The figure shows three views and two pictorial views of one solid part (mm, origin at its lowest corner). Answer the questions. A direction names the side the tool comes from. Coordinates: 2 decimals unless noted, no trailing zeros. Loops run counter-clockwise (first coordinate to the right, second up) from the corner with the lowest first, then second, coordinate; pieces in that order, holes last. Notation, with made-up numbers: (-8.5, 81) -> (36.5, 81) arc R9 ccw to (36.5, 86) -> close; hole circle Ø7 at (-24.75, -0.5). An arc over 180 degrees is marked (long way). Answer in a Markdown table with one row per item.
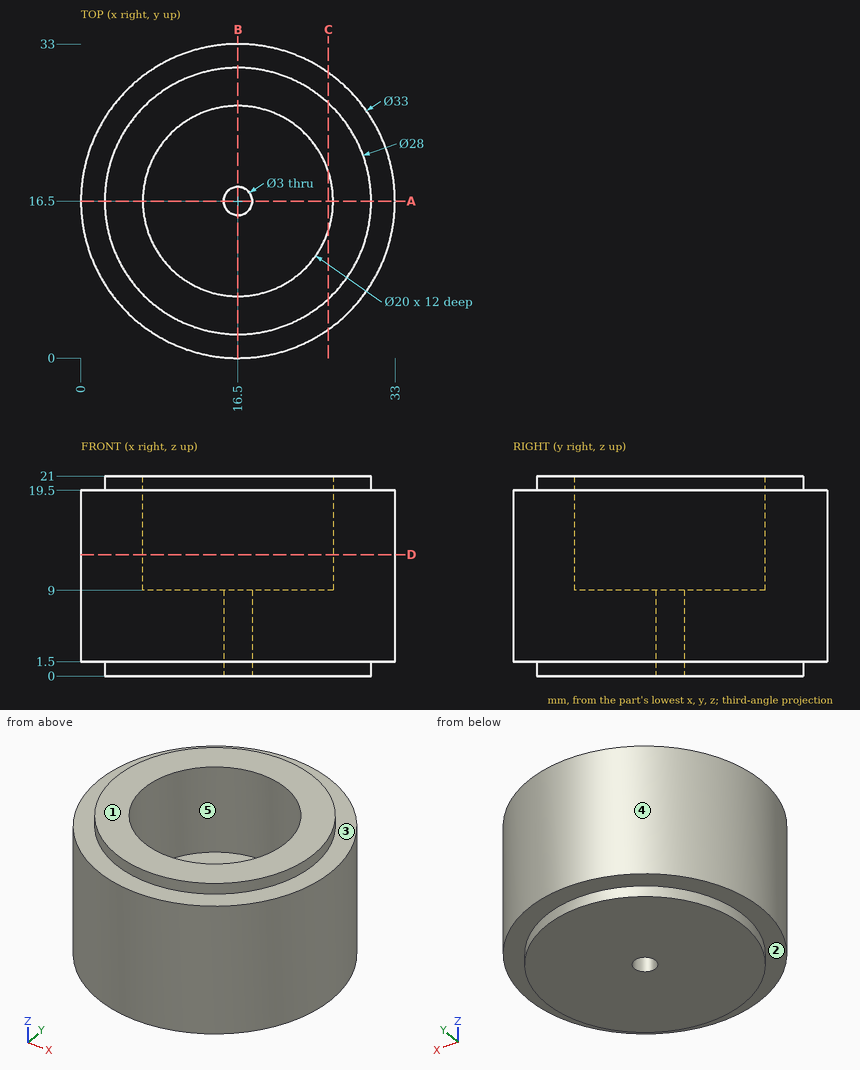
Item 1: Determine the mould class of the marked faces 3, 4 and 5 for opening direction X: +X half, -X half, draft (parallel to the pull), parting line (faces both ways), or undercut.
Findings below:
| item | result |
|---|---|
| face 3 | draft |
| face 4 | parting line |
| face 5 | undercut |
Item 2: A tool of negligible diameter and unlimited length cuts with its end or side. For the marked faces 1 and 2, from which of +Z, -Z, +X, -X, +Y, -Y can it reach the whole face along a straight path? Write none if from no direction.
Findings below:
| item | result |
|---|---|
| face 1 | +Z, +X, -X, +Y, -Y |
| face 2 | -Z |
Item 3: A cutting plane is placed at A-A, the plane y = 16.5. Determine the outline of the cut face in (x, z).
Findings below:
| item | result |
|---|---|
| outline | (0, 1.5) -> (2.5, 1.5) -> (2.5, 0) -> (15, 0) -> (15, 9) -> (6.5, 9) -> (6.5, 21) -> (2.5, 21) -> (2.5, 19.5) -> (0, 19.5) -> close; (18, 0) -> (30.5, 0) -> (30.5, 1.5) -> (33, 1.5) -> (33, 19.5) -> (30.5, 19.5) -> (30.5, 21) -> (26.5, 21) -> (26.5, 9) -> (18, 9) -> close |
Item 4: Flat-ended cylindrical pins translate along their axes: pin 1 Ø5 at (x, z) = (29.5, 8) entering from +Y; pin 2 Ø5 at (x, z) = (24.5, 3) entering from +Y; pin 3 Ø3 at (x, z) = (28.5, 7) entering from -Y. Find the tip coordinate at first contact, or state that the pin passes through.
Findings below:
| item | result |
|---|---|
| pin 1 | stops at y = 29.23 |
| pin 2 | stops at y = 32.06 |
| pin 3 | stops at y = 3.77 |
Item 5: A cutting plane is placed at C-C, the plane x = 26. Determine the outline of the cut face in (y, z).
Findings below:
| item | result |
|---|---|
| outline | (3.01, 1.5) -> (6.22, 1.5) -> (6.22, 0) -> (26.78, 0) -> (26.78, 1.5) -> (29.99, 1.5) -> (29.99, 19.5) -> (26.78, 19.5) -> (26.78, 21) -> (19.62, 21) -> (19.62, 9) -> (13.38, 9) -> (13.38, 21) -> (6.22, 21) -> (6.22, 19.5) -> (3.01, 19.5) -> close |
Item 6: A cutting plane is placed at D-D, the plane z = 12.75. Determine the outline of the cut face in (x, y).
Findings below:
| item | result |
|---|---|
| outline | circle Ø33 at (16.5, 16.5); hole circle Ø20 at (16.5, 16.5) |
Item 7: Find the intervals of material crossed by probe 1 along Y at (x, z) = (16.5, 5.5); probe 2 along Y at (x, z) = (16.5, 14.75); probe 3 along Z at (x, y) = (2.5, 23.5), in increasing order.
Findings below:
| item | result |
|---|---|
| probe 1 | y = 0 to 15, 18 to 33 |
| probe 2 | y = 0 to 6.5, 26.5 to 33 |
| probe 3 | z = 1.5 to 19.5 |
